from build123d import *

# Parameters (mm, degrees)
F0_R     = 1.5
F0_R_2   = 11
F1_DEPTH = 4


with BuildPart() as f1:
    # F0 (on Top) → F1 (new body)
    with BuildSketch(Plane.XY):
        with BuildLine():
            ThreePointArc((-21, -15.5), (-19.389087, -19.389087), (-15.5, -21))
            Line((-15.5, -21), (15.5, -21))
            ThreePointArc((15.5, -21), (19.389087, -19.389087), (21, -15.5))
            Line((21, -15.5), (21, 15.5))
            Line((21, 15.5), (26.075443, 18.580565))
            ThreePointArc((26.075443, 18.580565), (27.852125, 23.077557), (24, 26))
            Line((24, 26), (-24, 26))
            ThreePointArc((-24, 26), (-27.852125, 23.077557), (-26.075443, 18.580565))
            Line((-26.075443, 18.580565), (-21, 15.5))
            Line((-21, 15.5), (-21, -15.5))
        make_face()
        with Locations((-15.5, -15.5)):
            Circle(F0_R, mode=Mode.SUBTRACT)
        with Locations((15.5, -15.5)):
            Circle(F0_R, mode=Mode.SUBTRACT)
        Circle(F0_R_2, mode=Mode.SUBTRACT)
        with Locations((-15.5, 15.5)):
            Circle(F0_R, mode=Mode.SUBTRACT)
        with Locations((-24, 22)):
            Circle(F0_R, mode=Mode.SUBTRACT)
        with Locations((15.5, 15.5)):
            Circle(F0_R, mode=Mode.SUBTRACT)
        with Locations((24, 22)):
            Circle(F0_R, mode=Mode.SUBTRACT)
    extrude(amount=F1_DEPTH)


solid = f1.part
Part model, mm, in its own coordinate system. A direction names the side the tool comes from. Give positions to 0.01 mm unless a question says otherwise; leave off trailing zeros. Loops run counter-clockwise (first coordinate to the right, second up) from the corner with the lowest first, then second, coordinate; pieces in that order, holes last. Notation, with made-up numbers: (48, 24) -> (93, 24) arc R25 cw to (93, 41) -> close; hole circle Ø7 at (-10, 11). An arc over 180 degrees is marked (long way). Write each question's results on one line, items separated by ' | '. Start each with the question number.
Q1. Band-saw the part on B-B on x = -2. List the corners of the cut face in (y, z), plus the area to 3 significant figures.
Q2. Band-saw the part on D-D on y = 6. List the corners of the cut face in (x, z), plus the area to 3 significant figures.
Q3. Band-saw the part on C-C on z = 0.65. List the corners of the cut face in (x, y), plus the area to 3 significant figures.
Q4. Wall check: L1, parallel to Y at x = 15.5, z = 2.1; L2, parallel to X at y = -16, z = 3.45; L3, parallel to X at y = 16, z = 2.05. Give the ranges that are in metal, low to high.
Q5. Band-saw the part on A-A on y = 22. List the corners of the cut face in (x, z).
Q6. Pin check, flat tips, straight feed: P1, Ø2.5, axis at x = 24, y = 22, coming from the +Z side; P2, Ø1.5, axis at y = -14, z = 1, coming from the +X side; P3, Ø1, axis at x = -21, z = 1, coming from the -Y side; P4, Ø2, axis at y = -2, z = 3.5, coming from the -X side. Stop position of each tip, or through.
Q7. Which spindle directions (+Z, -Z, +X, -X, +Y, -Y) get a long thin tool onto all of the face, cutting with end or side? Do faces 4 (the face through (-2.38, -10.74, 1.97)), 5 (the face through (-21, 0, 2)). Say none if no direction does.
Q8. Pull direction X, two halves, no side cores. Call faces 1 (the face through (-23.57, 17.06, 1.97)), 2 (the face through (21, 0, 2)), 3 (the face through (-17, 15.57, 1.97)): +X half, -X half, draft (parallel to the pull), parting line (faces both ways), or undercut.
Results are:
1) outline: (-21, 0) -> (-10.82, 0) -> (-10.82, 4) -> (-21, 4) -> close; (10.82, 0) -> (26, 0) -> (26, 4) -> (10.82, 4) -> close | area: 101 mm²
2) outline: (-21, 0) -> (-9.22, 0) -> (-9.22, 4) -> (-21, 4) -> close; (9.22, 0) -> (21, 0) -> (21, 4) -> (9.22, 4) -> close | area: 94.2 mm²
3) outline: (-26.08, 18.58) -> (-21, 15.5) -> (-21, -15.5) arc R5.5 ccw to (-15.5, -21) -> (15.5, -21) arc R5.5 ccw to (21, -15.5) -> (21, 15.5) -> (26.08, 18.58) arc R4 ccw to (24, 26) -> (-24, 26) arc R4 ccw to start; hole circle Ø3 at (-24, 22); hole circle Ø3 at (-15.5, -15.5); hole circle Ø3 at (-15.5, 15.5); hole circle Ø22 at (0, 0); hole circle Ø3 at (15.5, -15.5); hole circle Ø3 at (15.5, 15.5); hole circle Ø3 at (24, 22) | area: 1,650 mm²
4) L1: y = -21 to -17, -14 to 14, 17 to 26 | L2: x = -20.98 to -16.91, -14.09 to 14.09, 16.91 to 20.98 | L3: x = -21.82 to -16.91, -14.09 to 14.09, 16.91 to 21.82
5) outline: (-28, 0) -> (-25.5, 0) -> (-25.5, 4) -> (-28, 4) -> close; (-22.5, 0) -> (22.5, 0) -> (22.5, 4) -> (-22.5, 4) -> close; (25.5, 0) -> (28, 0) -> (28, 4) -> (25.5, 4) -> close
6) P1: passes through | P2: stops at x = 21 | P3: stops at y = -17.79 | P4: stops at x = -21
7) face 4: +Z, -Z | face 5: +Z, -Z, -X, -Y
8) face 1: -X half | face 2: +X half | face 3: undercut
